Part model, mm, in its own coordinate system. Face numbers are marked on the shaded views. A direction names the side the tool comes from. Give positions to 0.01 mm unless a question says otherwise; leave off trailing zeros. Order: outer loops, then holes, each group sorted by start corner. A loop starts at its lowest first (then second) coordinate and runs counter-clockwise, first axis right, second up. Notation, with made-up numbers: (-1, -26.75) - (39, -26.75) arc R33 cw to (39, 1.25) - close; hole circle Ø10 at (54.25, 67). An arc over 180 degrees is marked (long way). One line per item, written item: value.
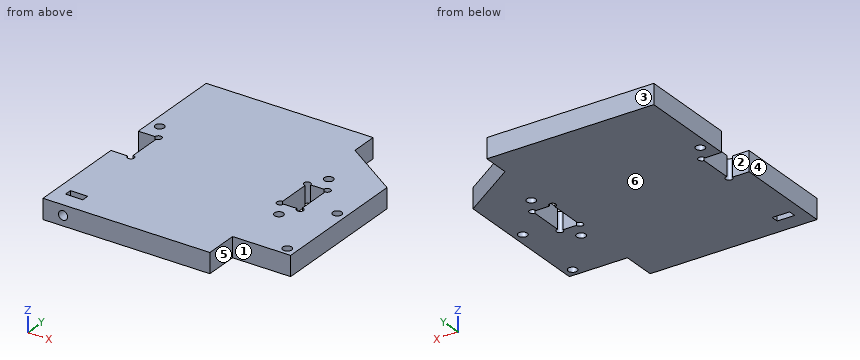
Autodesk Inventor part; units mm, degrees
ref_plane "YZ Plane" through (0, 0, 0) normal (1, 0, 0) x (0, 1, 0)
ref_plane "XZ Plane" through (0, 0, 0) normal (0, 1, 0) x (-1, 0, 0)
ref_plane "XY Plane" through (0, 0, 0) normal (0, 0, 1) x (1, 0, 0)
ref_plane "작업 평면1" through (0, 0, 0) normal (0, 0, 1) x (1, 0, 0)
sketch "스케치1" plane through (0, 0, 0) normal (0, 0, 1) x (1, 0, 0)
  arc A0 (20.1, 4.5766) -> (19.5808, 6.2636) centre (17.1, 4.5766) ccw
  line L0 (19.5808, 6.2636) -> (15.5953, 12.1246)
  arc A1 (15.5953, 12.1246) -> (13.9414, 13) centre (13.9414, 11) ccw
  line L1 (13, 13) -> (13.9414, 13)
  arc A2 (14.5, 11.5) -> (13, 13) centre (13, 11.5) ccw
  line L2 (14.5, -41.5) -> (14.5, 11.5)
  arc A3 (13.5, -42.5) -> (14.5, -41.5) centre (13.5, -41.5) ccw
  line L3 (-13.5, -42.5) -> (13.5, -42.5)
  arc A4 (-14.5, -41.5) -> (-13.5, -42.5) centre (-13.5, -41.5) ccw
  line L4 (-14.5, 11.5) -> (-14.5, -41.5)
  arc A5 (-13, 13) -> (-14.5, 11.5) centre (-13, 11.5) ccw
  line L5 (-13.9414, 13) -> (-13, 13)
  arc A6 (-13.9414, 13) -> (-15.5953, 12.1246) centre (-13.9414, 11) ccw
  line L6 (-15.5953, 12.1246) -> (-19.5808, 6.2636)
  arc A7 (-19.5808, 6.2636) -> (-20.1, 4.5766) centre (-17.1, 4.5766) ccw
  line L7 (-20.1, 4.5766) -> (-20.1, -39.6766)
  arc A8 (-20.1, -39.6766) -> (-19.5808, -41.3636) centre (-17.1, -39.6766) ccw
  line L8 (-19.5808, -41.3636) -> (-15.8929, -46.7869)
  arc A9 (-15.8929, -46.7869) -> (-13.4121, -48.1) centre (-13.4121, -45.1) ccw
  line L9 (-13.4121, -48.1) -> (13.4121, -48.1)
  arc A10 (13.4121, -48.1) -> (15.8929, -46.7869) centre (13.4121, -45.1) ccw
  line L10 (15.8929, -46.7869) -> (19.5808, -41.3636)
  arc A11 (19.5808, -41.3636) -> (20.1, -39.6766) centre (17.1, -39.6766) ccw
  line L11 (20.1, -39.6766) -> (20.1, 4.5766)
  circle A12 centre (-17.3, 4) radius 1.35
  circle A13 centre (-17.3, -18) radius 1.35
  circle A14 centre (-11, -45.3) radius 1.35
  circle A15 centre (17.3, 4) radius 1.35
  circle A16 centre (17.3, -18) radius 1.35
  circle A17 centre (11, -45.3) radius 1.35
  circle A18 centre (-17.3, -40) radius 1.35
  circle A19 centre (17.3, -40) radius 1.35
  arc A20 (-14.6, -41.5) -> (-13.5, -42.6) centre (-13.5, -41.5) ccw
  line L12 (-13.5, -42.6) -> (13.5, -42.6)
  arc A21 (13.5, -42.6) -> (14.6, -41.5) centre (13.5, -41.5) ccw
  line L13 (14.6, -41.5) -> (14.6, 11.5)
  arc A22 (14.6, 11.5) -> (12.2254, 12.9) centre (13, 11.5) ccw
  line L14 (12.2254, 12.9) -> (13.9414, 12.9)
  arc A23 (15.5126, 12.0684) -> (13.9414, 12.9) centre (13.9414, 11) ccw
  line L15 (15.5126, 12.0684) -> (19.4981, 6.2073)
  arc A24 (20, 4.5766) -> (19.4981, 6.2073) centre (17.1, 4.5766) ccw
  line L16 (20, 4.5766) -> (20, -39.6766)
  arc A25 (19.4981, -41.3073) -> (20, -39.6766) centre (17.1, -39.6766) ccw
  line L17 (19.4981, -41.3073) -> (15.8102, -46.7307)
  arc A26 (13.4121, -48) -> (15.8102, -46.7307) centre (13.4121, -45.1) ccw
  line L18 (13.4121, -48) -> (-13.4121, -48)
  arc A27 (-15.8102, -46.7307) -> (-13.4121, -48) centre (-13.4121, -45.1) ccw
  line L19 (-15.8102, -46.7307) -> (-18.6871, -42.5)
  line L20 (-19.4981, 6.2073) -> (-15.5126, 12.0684)
  arc A28 (-13.9414, 12.9) -> (-15.5126, 12.0684) centre (-13.9414, 11) ccw
  line L21 (-13.9414, 12.9) -> (-12.2254, 12.9)
  arc A29 (-12.2254, 12.9) -> (-14.6, 11.5) centre (-13, 11.5) ccw
  line L22 (-14.6, 11.5) -> (-14.6, -41.5)
  line L23 (-14.6, 11.5) -> (-20, 11.5)
  line L24 (-20, -42.5) -> (-14.6, -42.5)
  line L25 (-14.6, -42.5) -> (-14.6, 11.5)
  line L26 (-20, 11.5) -> (-32, 11.5)
  line L27 (-32, -42.5) -> (-20, -42.5)
  circle A30 centre (-17.3, 4) radius 1.35
  circle A31 centre (-17.3, -18) radius 1.35
  circle A32 centre (-17.3, -40) radius 1.35
  line L28 (-32, -9.5) -> (-26, -9.5)
  line L29 (-26, -9.5) -> (-26, -21.5)
  line L30 (-26, -21.5) -> (-32, -21.5)
  line L31 (-32, 11.5) -> (-32, -9.5)
  line L32 (-32, -21.5) -> (-32, -42.5)
  circle A33 centre (-29, -4.5) radius 1.35
  circle A34 centre (-29, -26.5) radius 1.35
  point P0 (0, 0)
  dimension "d0" = 0.1
  dimension "d2" = 2.7
  dimension "d3" = 2.7
  dimension "d4" = 2.7
  dimension "d5" = 12
  dimension "d6" = 2.7
  dimension "d7" = 2.7
extrude "돌출1" add sketch "스케치1" along normal blind 6 contours L24 L27 L32 L30 L29 L28 L31 L26 L23 L6 A7 L7 A8 L8 | L8 A8 L7 A7 L6 L23 L22 L25 L24
sketch "스케치2" plane through (-32, -42.5, 0) normal (-1, 0, 0) x (0, 0, 1)
  line L0 (0, 62) -> (6, 62)
  line L1 (6, 62) -> (6, -10)
  line L2 (6, -10) -> (0, -10)
  line L3 (0, -10) -> (0, 62)
  point P0 (0, 42.5)
  dimension "d10" = 6
  dimension "d11" = 72
extrude "돌출2" add sketch "스케치2" along normal blind 50
sketch "스케치3" plane through (0, 0, 6) normal (0, 0, 1) x (1, 0, 0)
  line L0 (-32, -42.5) -> (-14.6, -42.5)
  line L1 (-14.6, -42.5) -> (-14.6, 11.5)
  line L2 (-14.6, 11.5) -> (-32, 11.5)
  line L3 (-32, 11.5) -> (-32, 19.5)
  line L4 (-32, 19.5) -> (-82, 19.5)
  line L5 (-82, -52.5) -> (-82, 19.5)
  line L6 (-32, -52.5) -> (-82, -52.5)
  line L7 (-32, -52.5) -> (-32, -42.5)
  line L8 (-32, -21.5) -> (-32, -9.5)
  line L9 (-32, -9.5) -> (-26, -9.5)
  line L10 (-26, -9.5) -> (-26, -21.5)
  line L11 (-26, -21.5) -> (-32, -21.5)
  circle A0 centre (-17.3, -18) radius 1.35
  circle A1 centre (-17.3, 4) radius 1.35
  circle A2 centre (-17.3, -40) radius 1.35
  circle A3 centre (-29, -26.5) radius 1.35
  circle A4 centre (-29, -4.5) radius 1.35
  line L12 (-14.6, 0) -> (-32, 11.5)
  line L13 (-32, 11.5) -> (-14.6, 11.5)
  point P0 (0, 0)
extrude "돌출3" cut sketch "스케치3" against normal blind 50 contours L12 L2 L1
sketch "스케치5" plane through (-82, -42.5, 0) normal (-1, 0, 0) x (0, 0, 1)
  line L0 (-2.9941, 20.5626) -> (2.9941, 31.4374) construction
  line L1 (2.9941, 20.5626) -> (-2.9941, 31.4374) construction
  line L2 (0, 20) -> (0, 32)
  line L3 (6, 32) -> (6, 20)
  line L4 (6, 20) -> (0, 32) construction
  line L5 (0, 20) -> (6, 32) construction
  line L6 (6.025, 19.95) -> (-0.025, 19.95)
  line L7 (-0.025, 19.95) -> (-0.025, 32.05)
  line L8 (-0.025, 32.05) -> (6.025, 32.05)
  line L9 (6.025, 32.05) -> (6.025, 19.95)
  line L10 (6.025, 19.95) -> (-0.025, 32.05) construction
  line L11 (-0.025, 19.95) -> (6.025, 32.05) construction
  point P0 (0, 42.5)
  point P1 (0, 26)
  point P2 (3, 26)
  dimension "d16" = 6
  dimension "d17" = 12
  dimension "d18" = 12.1
extrude "돌출4" cut sketch "스케치5" against normal blind 6
sketch "스케치6" plane through (0, 0, 6) normal (0, 0, 1) x (1, 0, 0)
  line L0 (-76, -10.45) -> (-76, -22.55)
  line L1 (-82, -10.45) -> (-76, -10.45)
  line L2 (-76, -22.55) -> (-82, -22.55)
  circle A0 centre (-79, -5.45) radius 1.35
  point P0 (0, 0)
  dimension "d21" = 2.7
extrude "돌출5" cut sketch "스케치6" against normal blind 6
sketch "스케치7" plane through (-32, -52.5, 0) normal (0, -1, 0) x (1, 0, 0)
  line L0 (0, 0) -> (0, 6)
  line L1 (0, 6) -> (-50, 6)
  line L2 (-50, 0) -> (-50, 6)
  line L3 (0, 0) -> (-50, 0)
  circle A0 centre (-44, 3) radius 1.35
  point P0 (32, 0)
  dimension "d24" = 2.7
extrude "돌출6" cut sketch "스케치7" against normal blind 20 contours A0
sketch "스케치8" plane through (0, 0, 6) normal (0, 0, 1) x (1, 0, 0)
  circle A0 centre (-79, -5.45) radius 1.35
  line L0 (-76, -22.55) -> (-82, -22.55)
  line L1 (-82, -52.5) -> (-82, -22.55)
  line L2 (-32, -52.5) -> (-82, -52.5)
  line L3 (-32, -52.5) -> (-32, -42.5)
  line L4 (-32, -42.5) -> (-14.6, -42.5)
  line L5 (-14.6, -42.5) -> (-14.6, 0)
  line L6 (-14.6, 0) -> (-32, 11.5)
  line L7 (-32, 11.5) -> (-32, 19.5)
  line L8 (-32, 19.5) -> (-82, 19.5)
  line L9 (-82, -10.45) -> (-82, 19.5)
  line L10 (-82, -10.45) -> (-76, -10.45)
  line L11 (-76, -10.45) -> (-76, -22.55)
  line L12 (-32, -21.5) -> (-32, -9.5)
  line L13 (-32, -9.5) -> (-26, -9.5)
  line L14 (-26, -9.5) -> (-26, -21.5)
  line L15 (-26, -21.5) -> (-32, -21.5)
  circle A1 centre (-17.3, -18) radius 1.35
  circle A2 centre (-17.3, -40) radius 1.35
  circle A3 centre (-29, -26.5) radius 1.35
  circle A4 centre (-29, -4.5) radius 1.35
  line L16 (-73.4, -45.4) -> (-78.6, -45.4)
  line L17 (-78.6, -45.4) -> (-78.6, -47.6)
  line L18 (-78.6, -47.6) -> (-73.4, -47.6)
  line L19 (-73.4, -47.6) -> (-73.4, -45.4)
  line L20 (-73.4, -45.4) -> (-78.6, -47.6) construction
  line L21 (-78.6, -45.4) -> (-73.4, -47.6) construction
  point P0 (0, 0)
  point P1 (-76, -46.5)
  dimension "d27" = 5.2
  dimension "d28" = 2.2
extrude "돌출7" cut sketch "스케치8" against normal blind 20 contours L19 L18 L17 L16
sketch "스케치9" plane through (0, 0, 6) normal (0, 0, 1) x (1, 0, 0)
  line L0 (-76, -10.45) -> (-76, -22.55)
  line L1 (-82, -10.45) -> (-76, -10.45)
  line L2 (-76, -22.55) -> (-82, -22.55)
  line L3 (-32, -21.5) -> (-32, -9.5)
  line L4 (-32, -9.5) -> (-26, -9.5)
  line L5 (-26, -9.5) -> (-26, -21.5)
  line L6 (-26, -21.5) -> (-32, -21.5)
  circle A0 centre (-76, -10.45) radius 1
  circle A1 centre (-76, -22.55) radius 1
  circle A2 centre (-32, -9.5) radius 1
  circle A3 centre (-26, -9.5) radius 1
  circle A4 centre (-26, -21.5) radius 1
  circle A5 centre (-32, -21.5) radius 1
  point P0 (0, 0)
  dimension "d31" = 2
  dimension "d32" = 2
  dimension "d33" = 2
  dimension "d34" = 2
  dimension "d35" = 2
  dimension "d36" = 2
extrude "돌출8" cut sketch "스케치9" against normal blind 10 contours L1 A0 L0 | L0 A0 L1 | A1 L2 L0 | L0 L2 A1 | L6 A5 L3 | L3 A5 L6 | A2 L4 L3 | L3 L4 A2 | A4 L5 L6 | L6 L5 A4 | A3 L5 L4 | L4 L5 A3
properties part number "side of head" material "PMMA 플라스틱"
1) Drop flat-ended pins along their axis: P1, Ø1.2, axis at x = -26, y = -21.5, coming from the +Z side; P2, Ø4.5, axis at x = -17.3, y = -40, coming from the -Z side; P3, Ø3, axis at x = -29.5, z = 2.5, coming from the -Y side; P4, Ø2, axis at x = -28.5, z = 2, coming from the +Y side. Give the stop position or say it passes through.
Answer:
P1: passes through
P2: stops at z = 0
P3: stops at y = -42.5
P4: stops at y = 9.85
2) Slice it at B-B on y = -18. Write the cut outline in (x, z).
Answer:
outline: (-76, 0) - (-32, 0) - (-32, 6) - (-76, 6) - close; (-26, 0) - (-18.65, 0) - (-18.65, 6) - (-26, 6) - close; (-15.95, 0) - (-14.6, 0) - (-14.6, 6) - (-15.95, 6) - close
3) Wall check: line 1 along Z through (x, y) = (-76, -50.15); line 2 along Y through (x, z) = (-29, 2.8); line 3 along X through (y, z) = (-16, 4.8). Give the ranges that are in metal, low to high. Write a range as [from, to].
Answer:
line 1: z = [0, 1.65], [4.35, 6]
line 2: y = [-42.5, -27.85], [-25.15, -21.5], [-9.5, -5.85], [-3.15, 9.52]
line 3: x = [-76, -32], [-26, -14.6]
4) Two-plate mould, pull along Y, no slides. Class the marked faces 1, 2, 3 and 4: pulls with the +Y half, pulls with the -Y half, needs draft (parallel to the pull), parting line crosses it, or undercut.
Answer:
face 1: pulls with the -Y half
face 2: undercut
face 3: pulls with the +Y half
face 4: needs draft
5) Slice it at D-D on x = -29. Write the cut outline in (y, z).
Answer:
outline: (-42.5, 0) - (-27.85, 0) - (-27.85, 6) - (-42.5, 6) - close; (-25.15, 0) - (-21.5, 0) - (-21.5, 6) - (-25.15, 6) - close; (-9.5, 0) - (-5.85, 0) - (-5.85, 6) - (-9.5, 6) - close; (-3.15, 0) - (9.52, 0) - (9.52, 6) - (-3.15, 6) - close
6) Slice it at A-A on y = -40. Write the cut outline in (x, z), then the cut area to 3 significant figures.
Answer:
outline: (-82, 0) - (-18.65, 0) - (-18.65, 6) - (-82, 6) - close; (-15.95, 0) - (-14.6, 0) - (-14.6, 6) - (-15.95, 6) - close; hole circle Ø2.7 at (-76, 3)
area: 382 mm2
7) Which spindle directions (+Z, -Z, +X, -X, +Y, -Y) get a long thin tool onto all of the face, cutting with end or side? Do the marked faces 5 and 6. Say none if no direction does.
Answer:
face 5: +Z, -Z, +X, -Y
face 6: -Z, +X, -X, +Y, -Y
8) Slice it at C-C on x = -17.3. Write the cut outline in (y, z), then the cut area to 3 significant figures.
Answer:
outline: (-42.5, 0) - (-41.35, 0) - (-41.35, 6) - (-42.5, 6) - close; (-38.65, 0) - (-19.35, 0) - (-19.35, 6) - (-38.65, 6) - close; (-16.65, 0) - (1.78, 0) - (1.78, 6) - (-16.65, 6) - close
area: 233 mm2
